The model under review builds one solid part; all positions refer to its coordinate system, in mm. Face numbers are marked on the shaded views. Give positions to 0.01 mm unless a question says otherwise; leave off trailing zeros. Loops run counter-clockwise (first coordinate to the right, second up) from the corner with the lowest first, then second, coordinate; pieces in that order, holes last. Notation, with made-up numbers: M 70,-23 L 90,-23 A17 ccw 90,-7 Z; hole C 30.5,15.5 d6. An arc over 180 degrees is marked long. Return JSON: item names as keys, results as strings.
Autodesk Inventor part; units mm, degrees
ref_plane "YZ Plane" through (0, 0, 0) normal (1, 0, 0) x (0, 1, 0)
ref_plane "XZ Plane" through (0, 0, 0) normal (0, 1, 0) x (-1, 0, 0)
ref_plane "XY Plane" through (0, 0, 0) normal (0, 0, 1) x (1, 0, 0)
sketch "Sketch1" plane through (0, 0, 0) normal (0, 0, 1) x (1, 0, 0)
  line L0 (-89.1004, -3.8352) -> (336.0988, -78.8093)
  line L1 (336.0988, -75.5853) -> (336.0988, -78.8093)
  line L2 (336.0988, -75.5853) -> (-88.549, -0.7084)
  line L3 (-183.001, 111.8551) -> (-183.001, 183.0419)
  line L4 (-186.176, 183.0419) -> (-183.001, 183.0419)
  line L5 (-186.176, 183.0419) -> (-186.176, 111.8551)
  arc A0 (-186.176, 111.8551) -> (-89.1004, -3.8352) centre (-68.701, 111.8551) ccw
  arc A1 (-183.001, 111.8551) -> (-88.549, -0.7084) centre (-68.701, 111.8551) ccw
  point P0 (0, 0)
extrude "Extrusion1" add sketch "Sketch1" along normal blind 117.475
hole "Hole1" at (-186.176, 170.3419, 109.5375) direction (1, 0, 0) diameter 6.731 depth 25.4 tip angle 118
pattern_linear "Rectangular Pattern1" count 2 spacing 68.2625 along (0, 0, -1) of "Hole1"
hole "Hole2" at (323.5917, -76.6039, 109.5375) direction (0.1736482, 0.9848078, 0) diameter 6.731 depth 25.4 tip angle 118
pattern_linear "Rectangular Pattern2" count 2 spacing 368.3 along (-0.9848078, 0.1736482, 0) of "Hole2"
properties part number "GE-12086-02"
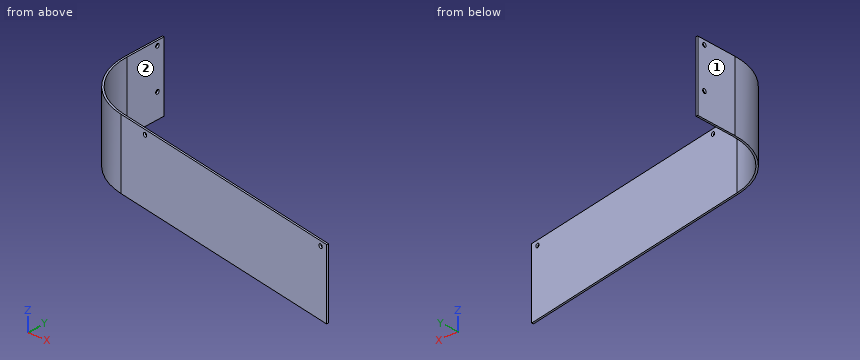
1) Wall thickness on L1, parallel to X at y = 158, z = 71; L2, parallel to Y at x = 86.5, z = 57; L3, parallel to Y at x = -61, z = 60.5: over which ranges is each line inside the solid? List them lowest first. Write a range as from..to.
From the geometry:
{"L1": "-186.18..-183", "L2": "-34.8..-31.57", "L3": "-8.79..-5.57"}
2) The part is to be moulded in two halves that separate along X. For the marked faces 1 and 2, say which applies: released by +X, released by -X, zero draft, split by the parting line, or undercut.
From the geometry:
{"face 1": "released by -X", "face 2": "released by +X"}
3) Insertion check: pin 1 (11 mm diameter, centred on y = 170.34, z = 41.28, fed in from +X); pin 2 (1 mm diameter, centred on y = 38.5, z = 22.5, fed in from +X); pin 3 (6 mm diameter, centred on x = -57.5, z = 51.5, fed in from +Y). Each pin has a flat end and moves straight along its axis. Give the tip position at first contact, or say it passes through.
From the geometry:
{"pin 1": "x = -183", "pin 2": "x = -155.94", "pin 3": "y = -5.65"}
4) Consider section C-C on x = -80.5. Write out the cut boundary in (y, z) (3 decimals), then the cut area to 3 significant figures.
From the geometry:
{"outline": "M -5.352,0 L -2.128,0 L -2.128,117.475 L -5.352,117.475 Z", "area": "379 mm²"}
5) Consider section A-A on z = 8.5. Write out the cut boundary in (x, y), then the cut area to 3 significant figures.
From the geometry:
{"outline": "M -186.18,111.86 A117.48 ccw -89.1,-3.84 L 336.1,-78.81 L 336.1,-75.59 L -88.55,-0.71 A114.3 cw -183,111.86 L -183,183.04 L -186.18,183.04 Z", "area": "2,110 mm²"}
6) Consider section B-B on y = 100.5. Write out the cut boundary in (x, z) (3 decimals), then the cut area to 3 significant figures.
From the geometry:
{"outline": "M -185.626,0 L -182.436,0 L -182.436,117.475 L -185.626,117.475 Z", "area": "375 mm²"}
